Could you check a few things on this model? Use its own coordinates, in mm. Give positions to 0.01 mm unless a question says otherwise; leave off trailing zeros. Write each loop counter-clockwise with the first axis right and the second up, starting at its lowest first coordinate (ties: lowest second). Pieces come first, ordered by that corner, then holes. Notation, with made-up numbers: M -23.75,79 L 28.25,79 A19 ccw 28.25,107 Z; hole C 13.25,18 d11. An arc over 180 degrees is marked long. Answer as a JSON object with one key per item and string values. Group by question number.
```python
from build123d import *


with BuildPart() as f1:
    # F0 (on Front) → F1 (revolve)
    with BuildSketch(Plane.XZ):
        Polygon((-41.275, 0), (-44.45, 0), (-44.45, -1.46647), (-44.45, -3.05397), (-44.45, -4.520439), (-44.45, -5.588), (-41.275, -5.588), align=None)
        Polygon((-44.45, -1.46647), (-44.45, 0), (-45.72, -0.733235), (-45.085, -1.833087), align=None)
        Polygon((-44.45, -4.520439), (-44.45, -3.05397), (-45.085, -3.420587), align=None)
    revolve(axis=Axis((0, 0, -1.429696), (0, 0, -1)))


solid = f1.part
```
1) I'm going to push flat-ended pins straight in: pin 1 (2 mm diameter, centred on x = -34.5, z = -1, fed in from -Y); pin 2 (2 mm diameter, centred on x = -31.5, z = -4, fed in from +Y); pin 3 (1 mm diameter, centred on x = 20, z = -4.5, fed in from +Y). Where does each tip first touch, or does it pass through?
2) Please list where these lines run through material, in increasing order: line 1 along Y through (x, z) = (0, -2.1) (3 decimals); line 2 along Y through (x, z) = (0, -3.45) (3 decimals); line 3 along Y through (x, z) = (0, -1.75) (3 decimals). Write a range as from..to.
3) We'd pull the mould along X, two halves only. Please class faces 1 (the flat face through (29.4, -29.4, 0)), 2 (the cylindrical face through (-42.397, 13.352, -2.271)), 3 (the cylindrical face through (-42.397, 13.352, -5.062)): released by +X, released by -X, zero draft, split by the parting line, or undercut.
4) If we section it at A-A, the plane x = 0: List the corners of the cut face in (y, z) for me (3 decimals).
Taken from the geometry:
{
 "1": {"pin 1": "y = -31.07", "pin 2": "y = 33.03", "pin 3": "y = 40.12"},
 "2": {"line 1": "-44.45..-41.275, 41.275..44.45", "line 2": "-45.068..-41.275, 41.275..45.068", "line 3": "-45.133..-44.941, -44.45..-41.275, 41.275..44.45, 44.941..45.133"},
 "3": {"face 1": "zero draft", "face 2": "undercut", "face 3": "split by the parting line"},
 "4": {"outline": "M -45.72,-0.733 L -45.085,-1.833 L -44.45,-1.466 L -44.45,-3.054 L -45.085,-3.421 L -44.45,-4.52 L -44.45,-5.588 L -41.275,-5.588 L -41.275,0 L -44.45,0 Z; M 41.275,-5.588 L 44.45,-5.588 L 44.45,-4.52 L 45.085,-3.421 L 44.45,-3.054 L 44.45,-1.466 L 45.085,-1.833 L 45.72,-0.733 L 44.45,0 L 41.275,0 Z"}
}
